Autodesk Inventor part; units mm, degrees
ref_plane "YZ Plane" through (0, 0, 0) normal (1, 0, 0) x (0, 1, 0)
ref_plane "XZ Plane" through (0, 0, 0) normal (0, 1, 0) x (-1, 0, 0)
ref_plane "XY Plane" through (0, 0, 0) normal (0, 0, 1) x (1, 0, 0)
sketch "Sketch1" plane through (0, 0, 0) normal (0, 1, 0) x (-1, 0, 0)
  circle A0 centre (0, 0) radius 10
  dimension "d0" = 20
extrude "Extrusion1" add sketch "Sketch1" along normal blind 1.5
sketch "Sketch2" plane through (0, 1.5, 0) normal (0, 1, 0) x (1, 0, 0)
  circle A0 centre (0, 0) radius 5.875
  dimension "d3" = 11.75
extrude "Extrusion2" cut sketch "Sketch2" against normal blind 1
sketch "Sketch3" plane through (0, 0.5, 0) normal (0, 1, 0) x (1, 0, 0)
  circle A0 centre (0, 0) radius 2
  dimension "d6" = 4
extrude "Extrusion3" cut sketch "Sketch3" against normal through all
properties part number "M3Bearing_Holder"
Could you check a few things on this model? Use its own coordinates, in mm. A direction names the side the tool comes from. Coordinates: 2 decimals unless noted, no trailing zeros. Write each loop counter-clockwise with the first axis right and the second up, starting at its lowest first coordinate (ties: lowest second). Pieces come first, ordered by that corner, then holes. Notation, with made-up numbers: (57.5, -21.5) - (83.5, -21.5) arc R14 ccw to (83.5, 1.5) - close; hole circle Ø11 at (19.5, 80.25). An arc over 180 degrees is marked (long way). Write item = value, one per line.
1) Suppose I cut it at D-D on z = -4.75. Please give me the cut outline in (x, y), plus the area to 3 significant figures.
Result set:
outline = (-8.8, 0) - (8.8, 0) - (8.8, 1.5) - (3.46, 1.5) - (3.46, 0.5) - (-3.46, 0.5) - (-3.46, 1.5) - (-8.8, 1.5) - close
area = 19.5 mm2
2) Please list where these lines run through material, in increasing order: line 1 (Z direction, x = 0, y = 1.15) (3 decimals); line 2 (Z direction, x = 0, y = 0.2); line 3 (Y direction, x = 3.25, z = -2.25). Write a range as [from, to].
Result set:
line_1 = [-10, -5.875], [5.875, 10]
line_2 = [-10, -2], [2, 10]
line_3 = [0, 0.5]
3) For faces 1 (the flat face through (0.1, 0, 2.4)), 2 (the flat face through (3, 0.5, 0)), which set-ups out of +Z, -Z, +X, -X, +Y, -Y let a thin tool reach every point of the face, with its end or its side?
Result set:
face_1 = +Z, -Z, +X, -X, -Y
face_2 = +Y
4) Suppose I cut it at B-B on z = -0.25. Please give me the cut outline in (x, y).
Result set:
outline = (-10, 0) - (-1.98, 0) - (-1.98, 0.5) - (-5.87, 0.5) - (-5.87, 1.5) - (-10, 1.5) - close; (1.98, 0) - (10, 0) - (10, 1.5) - (5.87, 1.5) - (5.87, 0.5) - (1.98, 0.5) - close
5) Suppose I cut it at C-C on y = 1.2. Please give me the cut outline in (x, z) (3 decimals).
Result set:
outline = circle Ø20 at (0, 0); hole circle Ø11.75 at (0, 0)
6) Suppose I cut it at A-A on x = 0. Please give me the cut outline in (y, z) (3 decimals).
Result set:
outline = (0, -10) - (1.5, -10) - (1.5, -5.875) - (0.5, -5.875) - (0.5, -2) - (0, -2) - close; (0, 2) - (0.5, 2) - (0.5, 5.875) - (1.5, 5.875) - (1.5, 10) - (0, 10) - close
7) Will this pin go through, and if not, where does the flat tip stop? pin 1 Ø3.5 at (x, z) = (0, 0) entering from +Y.
Result set:
pin_1 = through
8) We'd pull the mould along X, two halves only. Please class faces 3 (the flat face through (-4.3, 1.5, -4.3)), 4 (the cylindrical face through (2.17, 0.74, 9.76)), 5 (the cylindrical face through (5.604, 1.007, -1.765)), 6 (the cylindrical face through (-0.434, 0.254, 1.952)): +X half, -X half, draft (parallel to the pull), parting line (faces both ways), or undercut.
Result set:
face_3 = draft
face_4 = parting line
face_5 = undercut
face_6 = undercut
